The listing builds one solid part. Answer for the finished solid, in the listing's coordinates (mm). Face numbers are marked on the shaded views. A direction names the side the tool comes from. Coordinates: 2 decimals unless noted, no trailing zeros. Write each loop counter-clockwise with the first axis right and the second up, starting at its lowest first coordinate (ties: lowest second). Pieces come first, ordered by that corner, then holes. Notation, with made-up numbers: M 18.25,-24 L 40.25,-24 A20 cw 40.25,-18 Z; hole C 25,73.25 d5. An arc over 180 degrees is marked long. Write item = value, one per line. Start each with the question number.
```python
from build123d import *

# Parameters (mm, degrees)
SKETCH2_W           = 33
SKETCH2_H           = 33
SKETCH2_R           = 8.65
BOSS_EXTRUDE1_DEPTH = 8
SKETCH3_W           = 8
SKETCH3_H           = 26
BOSS_EXTRUDE2_DEPTH = 3
SKETCH4_W           = 26
SKETCH4_H           = 21
SKETCH4_R           = 8.1
BOSS_EXTRUDE3_DEPTH = 2.12
SKETCH5_R           = 1.5
BOSS_EXTRUDE4_DEPTH = 2
BOSS_EXTRUDE5_DEPTH = 6
SKETCH7_R           = 1.65
CUT_EXTRUDE1_DEPTH  = 10


with BuildPart() as part:
    # Sketch2 → Boss-Extrude1 (new body)
    with BuildSketch(Plane.XY):
        with Locations((16.5, 16.5)):
            Rectangle(SKETCH2_W, SKETCH2_H)
        with Locations((16.5, 16.5)):
            Circle(SKETCH2_R, mode=Mode.SUBTRACT)
    extrude(amount=BOSS_EXTRUDE1_DEPTH)

    # Sketch3 → Boss-Extrude2 (add)
    with BuildSketch(Plane(origin=(33, 0, 0), x_dir=(0, 0, -1), z_dir=(1, 0, 0))):
        with Locations((-4, 16)):
            Rectangle(SKETCH3_W, SKETCH3_H)
    extrude(amount=BOSS_EXTRUDE2_DEPTH)

    # Sketch4 → Boss-Extrude3 (add)
    with BuildSketch(Plane(origin=(16.5, 0, -16.5), x_dir=(0, 1, 0), z_dir=(0.707106781, 0, -0.707106781))):
        with Locations((16, 14.955844123)):
            Rectangle(SKETCH4_W, SKETCH4_H)
        with Locations((16, 14.955844123)):
            Circle(SKETCH4_R, mode=Mode.SUBTRACT)
    extrude(amount=BOSS_EXTRUDE3_DEPTH)

    # Sketch5 → Boss-Extrude4 (add)
    with BuildSketch(Plane.XY.offset(8)):
        with Locations((2.5, 30.5)):
            Circle(SKETCH5_R)
    extrude(amount=BOSS_EXTRUDE4_DEPTH)

    # Sketch6 → Boss-Extrude5 (add)
    with BuildSketch(Plane.XY.offset(10)):
        with BuildLine():
            Line((7.22, 0), (7.22, 7.823187296))
            ThreePointArc((7.22, 7.823187296), (10.728461041, 24.490588089), (27.694109386, 26))
            Line((27.694109386, 26), (33, 26))
            Line((33, 26), (33, 50))
            Line((33, 50), (0, 50))
            Line((0, 50), (0, 0))
            Line((0, 0), (7.22, 0))
        make_face()
    extrude(amount=BOSS_EXTRUDE5_DEPTH)

    # Sketch7 → Cut-Extrude1 (cut)
    with BuildSketch(Plane(origin=(0, 50, 0), x_dir=(1, 0, 0), z_dir=(0, 1, 0))):
        with Locations((6.77, -12.75)):
            Circle(SKETCH7_R)
        with Locations((26.2, -13.15)):
            Circle(SKETCH7_R)
    extrude(amount=-CUT_EXTRUDE1_DEPTH, mode=Mode.SUBTRACT)


solid = part.part
```
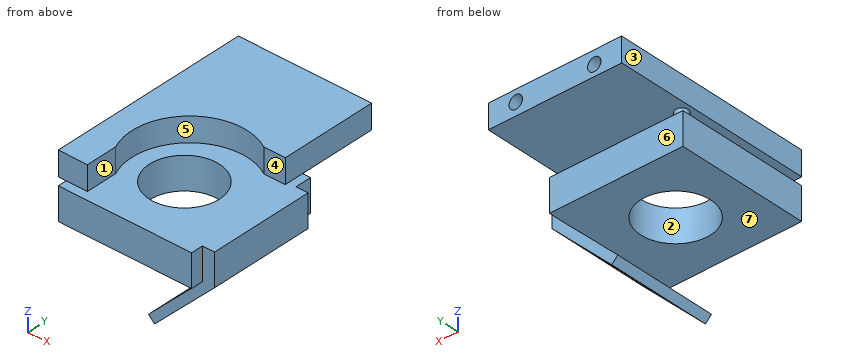
1. The part is cut by section D-D, the plane y = 30.5. Write down the section's boundary in (x, z).
2. For the marked faces 4, 5, 6 and 7, determine the directions among +Z, -Z, +X, -X, +Y, -Y from which every point of the face is accessible in a straight line to the end or side of a thin tool.
3. The part is cut by section A-A, the plane z = 4.5. Write down the section's boundary in (x, y).
4. The part is cut by section C-C, the plane x = 19. Write down the section's boundary in (y, z), and give its area (3 significant figures).
5. The part is cut by section B-B, the plane y = 23. Count the separate pieces of the cut face and the enclosed holes in it, and give its area (3 significant figures).
6. Each of these flat-tipped pins is pushed along its axis until it touches: pin 1 (5 mm diameter, centred on x = 23.5, y = 36.5, fed in from -Z); pin 2 (5 mm diameter, centred on x = 28, z = -4.5, fed in from +Y); pin 3 (3 mm diameter, centred on y = 34, z = 13.5, fed in from +X); pin 4 (3 mm diameter, centred on y = 30, z = 5.5, fed in from +X). Where does it stop, or does it pass through?
7. Straight lines are drawn through the part: L1, parallel to Z at x = 26, y = 47; L2, parallel to X at y = 16, z = 4; L3, parallel to Z at x = 6.77, y = 46. For each, find the intervals that lie inside material, in ascending order. Write a range as [from, to].
8. For a pull along X with two mould halves and no side action, classify the marked faces 1, 2 and 3 as pulls with the +X half, pulls with the -X half, needs draft (parallel to the pull), parting line crosses it, or undercut.
Solution:
q1.outline = M 0,0 L 33,0 L 33,8 L 4,8 L 4,10 L 33,10 L 33,16 L 0,16 L 0,10 L 1,10 L 1,8 L 0,8 Z
q2.face_4 = +Z, +X, -Y
q2.face_5 = +Z
q2.face_6 = -Z, +X, -X, +Y
q2.face_7 = -X, +Y, -Y
q3.outline = M 0,0 L 33,0 L 33,3 L 36,3 L 36,29 L 33,29 L 33,33 L 0,33 Z; hole C 16.5,16.5 d17.3
q4.outline = M 0,0 L 8.22,0 L 8.22,8 L 0,8 Z; M 24.78,0 L 33,0 L 33,8 L 24.78,8 Z; M 28.05,10 L 50,10 L 50,16 L 28.05,16 Z
q4.area = 263 mm^2
q5.separate_pieces = 4
q5.enclosed_holes = 0
q5.area = 277 mm^2
q6.pin_1 = 10
q6.pin_2 = 29
q6.pin_3 = 33
q6.pin_4 = 36
q7.L1 = [10, 11.51], [14.79, 16]
q7.L2 = [0, 7.86], [25.14, 36]
q7.L3 = [10, 11.1], [14.4, 16]
q8.face_1 = pulls with the +X half
q8.face_2 = undercut
q8.face_3 = pulls with the -X half
